from build123d import *

# Parameters (mm, degrees)
SKIZZE1_W                       = 6
SKIZZE1_H                       = 23.2
SKIZZE1_W_2                     = 1.7
SKIZZE1_H_2                     = 14
AUFSATZ_LINEAR_AUSTRAGEN1_DEPTH = 0.825
VERRUNDUNG2_R                   = 0.85


with BuildPart() as part:
    # Skizze1 → Aufsatz-Linear austragen1 (new, symmetric)
    with BuildSketch(Plane(origin=(0, 0, 0), x_dir=(1, 0, 0), z_dir=(0, 1, 0))):
        Rectangle(SKIZZE1_W, SKIZZE1_H)
        with Locations((0.15, 0)):
            Rectangle(SKIZZE1_W_2, SKIZZE1_H_2, mode=Mode.SUBTRACT)
    extrude(amount=AUFSATZ_LINEAR_AUSTRAGEN1_DEPTH, both=True)

    # Verrundung2
    verrundung2_edges = [part.edges().sort_by_distance(p)[0] for p in [
        (-0.7, 0, 7),
        (1, 0, 7),
        (1, 0, -7),
        (-0.7, 0, -7),
    ]]
    fillet(verrundung2_edges, radius=VERRUNDUNG2_R - 0.0001)  # a hair under: the kernel refuses the full size


solid = part.part
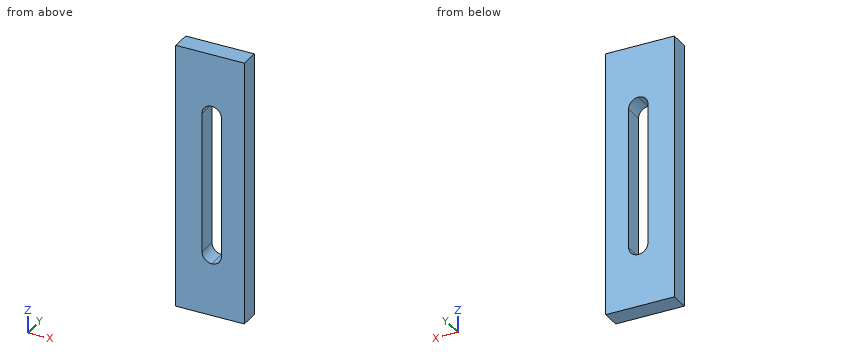
Can you work these out from the model? Positions are in its coordinate system, mm. Coordinates: 2 decimals unless noted, no trailing zeros. Order: outer loops, then holes, each group sorted by start corner. A loop starts at its lowest first (then second) coordinate and runs counter-clockwise, first axis right, second up. Notation, with made-up numbers: M 41,1.25 L 55,1.25 A23 ccw 55,36.25 Z; hole C 24.5,77 d9. An arc over 180 degrees is marked long. Write item = value, one per line.
(1) Suppose I cut it at B-B on z = 1. Please give me the cut outline in (x, y) (3 decimals), plus the area to 4 significant figures.
Results are:
outline = M -3,-0.825 L -0.7,-0.825 L -0.7,0.825 L -3,0.825 Z; M 1,-0.825 L 3,-0.825 L 3,0.825 L 1,0.825 Z
area = 7.095 mm2
(2) I need wall thicknesses on line 1 along X through (y, z) = (0.4, 3.25); line 2 along Z through (x, y) = (0.4, -0.45); line 3 along Z through (x, y) = (0.9, -0.2). Which ranges of each line are inside material? Lowest first, please. Write a range as [from, to].
Results are:
line_1 = [-3, -0.7], [1, 3]
line_2 = [-11.6, -6.96], [6.96, 11.6]
line_3 = [-11.6, -6.55], [6.55, 11.6]
(3) Suppose I cut it at C-C on x = 0.8. Please give me the cut outline in (y, z) (3 decimals).
Results are:
outline = M -0.825,-11.6 L 0.825,-11.6 L 0.825,-6.698 L -0.825,-6.698 Z; M -0.825,6.698 L 0.825,6.698 L 0.825,11.6 L -0.825,11.6 Z
